Part model, mm, in its own coordinate system. Face numbers are marked on the shaded views. A direction names the side the tool comes from. Give positions to 0.01 mm unless a question says otherwise; leave off trailing zeros. Order: outer loops, then holes, each group sorted by start corner. A loop starts at its lowest first (then second) coordinate and runs counter-clockwise, first axis right, second up. Notation, with made-up numbers: (25.25, 8.5) - (41.25, 8.5) arc R25 cw to (41.25, 31.5) - close; hole circle Ø7 at (24.25, 63). An arc over 180 degrees is marked (long way). Use a Markdown table: item, result. Add a question column.
from build123d import *

# Parameters (mm, degrees)
SKETCH1_W           = 41
SKETCH1_H           = 41
SKETCH1_R           = 1.75
SKETCH1_R_2         = 1.25
BOSS_EXTRUDE1_DEPTH = 2
SKETCH2_W           = 10
SKETCH2_H           = 10
SKETCH2_R           = 1.75
BOSS_EXTRUDE2_DEPTH = 30
FILLET1_R           = 5


with BuildPart() as part:
    # Sketch1 → Boss-Extrude1 (new body)
    with BuildSketch(Plane.XY):
        with Locations((-34.508333333, 4.35625)):
            Rectangle(SKETCH1_W, SKETCH1_H)
        with Locations((-50.008333333, 19.85625)):
            Circle(SKETCH1_R, mode=Mode.SUBTRACT)
        with Locations((-50.008333333, -11.14375)):
            Circle(SKETCH1_R, mode=Mode.SUBTRACT)
        with Locations((-19.008333333, -11.14375)):
            Circle(SKETCH1_R, mode=Mode.SUBTRACT)
        with Locations((-19.008333333, 19.85625)):
            Circle(SKETCH1_R, mode=Mode.SUBTRACT)
        with Locations((-34.508333333, 4.35625)):
            Circle(SKETCH1_R_2, mode=Mode.SUBTRACT)
    extrude(amount=BOSS_EXTRUDE1_DEPTH)

    # Sketch2 → Boss-Extrude2 (add)
    # profile 1 of 4: a face of its own
    with BuildSketch(Plane.XY.offset(2)):
        with Locations((-50.008333333, 19.85625)):
            Rectangle(SKETCH2_W, SKETCH2_H)
        with Locations((-50.008333333, 19.85625)):
            Circle(SKETCH2_R, mode=Mode.SUBTRACT)
    # profile 2 of 4: a face of its own
    with BuildSketch(Plane.XY.offset(2)):
        with Locations((-50.008333333, -11.14375)):
            Rectangle(SKETCH2_W, SKETCH2_H)
        with Locations((-50.008333333, -11.14375)):
            Circle(SKETCH2_R, mode=Mode.SUBTRACT)
    # profile 3 of 4: a face of its own
    with BuildSketch(Plane.XY.offset(2)):
        with Locations((-19.008333333, -11.14375)):
            Rectangle(SKETCH2_W, SKETCH2_H)
        with Locations((-19.008333333, -11.14375)):
            Circle(SKETCH2_R, mode=Mode.SUBTRACT)
    # profile 4 of 4: a face of its own
    with BuildSketch(Plane.XY.offset(2)):
        with Locations((-19.008333333, 19.85625)):
            Rectangle(SKETCH2_W, SKETCH2_H)
        with Locations((-19.008333333, 19.85625)):
            Circle(SKETCH2_R, mode=Mode.SUBTRACT)
    extrude(amount=BOSS_EXTRUDE2_DEPTH)

    # Fillet1
    fillet1_edges = [part.edges().sort_by_distance(p)[0] for p in [
        (-24.008333333, 24.85625, 17),
        (-24.008333333, -6.14375, 17),
        (-55.008333333, -6.14375, 17),
        (-55.008333333, 14.85625, 17),
        (-45.008333333, 24.85625, 17),
        (-45.008333333, -6.14375, 17),
        (-45.008333333, -16.14375, 17),
        (-24.008333333, -16.14375, 17),
        (-14.008333333, -6.14375, 17),
        (-14.008333333, 14.85625, 17),
        (-24.008333333, 14.85625, 17),
        (-45.008333333, 14.85625, 17),
        (-14.008333333, -16.14375, 16),
        (-14.008333333, 24.85625, 16),
        (-55.008333333, -16.14375, 16),
        (-55.008333333, 24.85625, 16),
    ]]
    fillet(fillet1_edges, radius=FILLET1_R - 0.0001)  # a hair under: the kernel refuses the full size


solid = part.part
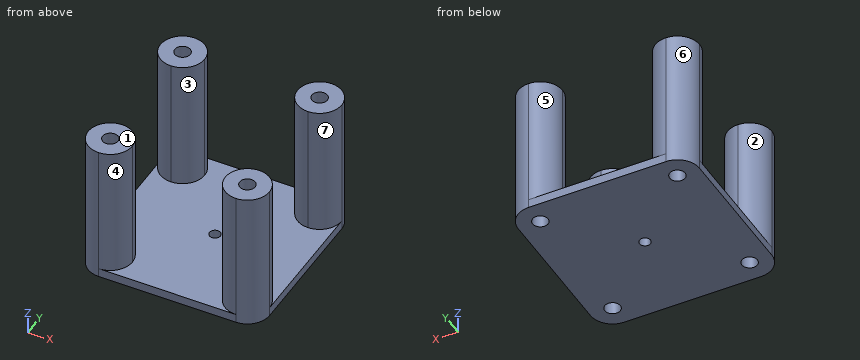
1. Cut at D-D (z = 25). State how many separate pieces and enclosed holes the cut face has, plus the area to 3 significant figures.
2. Tool access for the marked faces 1, 2, 3 and 4: list every direction of +Z, -Z, +X, -X, +Y, -Y with a clear straight run to the whole face (end or side of a thin tool).
3. Cut at C-C (x = -37.5). Write the cut outline in (y, z), plus the area to 3 significant figures.
4. Cut at A-A (x = -18). Write the cut outline in (y, z).
5. Pin check, flat tips, straight feed: P1, Ø2, axis at x = -36, y = 2.5, coming from the +Z side; P2, Ø6, axis at y = 13, z = 20, coming from the +X side; P3, Ø3, axis at x = -24.5, z = 25.5, coming from the +Y side. Stop position of each tip, or through.
6. Mould opens along X. For the marked faces 5, 6 and 7 say: released by +X, released by -X, zero draft, split by the parting line, or undercut.
7. Cut at B-B (y = 5). Write the cut outline in (x, z), plus the area to 3 significant figures.
8. Drill centre lines: probe 1 along Y at (x, z) = (-19, 24.5); probe 2 along X at (y, z) = (20, 5); probe 3 along X at (y, z) = (-10.5, 11.5). Where is each one in solid material? Low to high. Write a range as [from, to].
Responses:
| question | item | result |
|---|---|---|
| 1 | separate pieces | 4 |
| 1 | enclosed holes | 4 |
| 1 | area | 276 mm² |
| 2 | face 1 | +Z, +X, -X, +Y, -Y |
| 2 | face 2 | +Z, -X |
| 2 | face 3 | +Z |
| 2 | face 4 | +Z, -Y |
| 3 | outline | (-16.14, 0) - (24.86, 0) - (24.86, 2) - (-16.14, 2) - close |
| 3 | area | 82.0 mm² |
| 4 | outline | (-16.04, 0) - (-12.57, 0) - (-12.57, 32) - (-16.04, 32) - close; (-9.71, 0) - (18.43, 0) - (18.43, 32) - (14.96, 32) - (14.96, 2) - (-6.25, 2) - (-6.25, 32) - (-9.71, 32) - close; (21.29, 0) - (24.75, 0) - (24.75, 32) - (21.29, 32) - close |
| 5 | P1 | stops at z = 2 |
| 5 | P2 | stops at x = -15.83 |
| 5 | P3 | stops at y = 22.87 |
| 6 | face 5 | undercut |
| 6 | face 6 | released by -X |
| 6 | face 7 | released by +X |
| 7 | outline | (-55.01, 0) - (-35.58, 0) - (-35.58, 2) - (-55.01, 2) - close; (-33.44, 0) - (-14.01, 0) - (-14.01, 2) - (-33.44, 2) - close |
| 7 | area | 77.7 mm² |
| 8 | probe 1 | y = [-16.14, -12.89], [-9.39, -6.14], [14.86, 18.11], [21.61, 24.86] |
| 8 | probe 2 | x = [-55.01, -51.75], [-48.26, -45.01], [-24.01, -20.75], [-17.26, -14.01] |
| 8 | probe 3 | x = [-54.97, -51.64], [-48.38, -45.05], [-23.97, -20.64], [-17.38, -14.05] |
